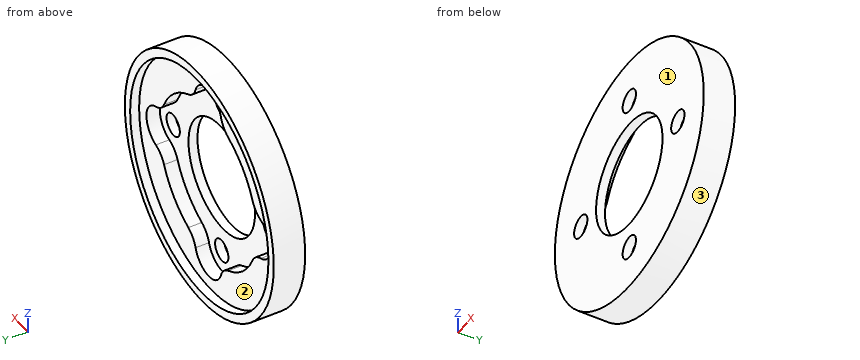
from build123d import *

# Parameters (mm, degrees)
SKETCH1_R           = 28
SKETCH1_R_2         = 12.5
SKETCH1_R_3         = 2.5
BOSS_EXTRUDE1_DEPTH = 5
SKETCH2_R           = 28
SKETCH2_R_2         = 26
BOSS_EXTRUDE2_DEPTH = 2
CUT_EXTRUDE1_DEPTH  = 3
FILLET1_R           = 5


with BuildPart() as part:
    # Sketch1 → Boss-Extrude1 (new body)
    with BuildSketch(Plane(origin=(0, 0, 0), x_dir=(1, 0, 0), z_dir=(0, 1, 0))):
        with Locations(Location((0, 0, 0), (0, 0, 270))):
            Circle(SKETCH1_R)
        with Locations(Location((0, 0, 0), (0, 0, 270))):
            Circle(SKETCH1_R_2, mode=Mode.SUBTRACT)
        with Locations(Location((18.25, 0, 0), (0, 0, 270))):
            Circle(SKETCH1_R_3, mode=Mode.SUBTRACT)
        with Locations(Location((0, -18.25, 0), (0, 0, 270))):
            Circle(SKETCH1_R_3, mode=Mode.SUBTRACT)
        with Locations(Location((-18.25, 0, 0), (0, 0, 270))):
            Circle(SKETCH1_R_3, mode=Mode.SUBTRACT)
        with Locations(Location((0, 18.25, 0), (0, 0, 270))):
            Circle(SKETCH1_R_3, mode=Mode.SUBTRACT)
    extrude(amount=BOSS_EXTRUDE1_DEPTH)

    # Sketch2 → Boss-Extrude2 (add)
    with BuildSketch(Plane(origin=(0, 5, 0), x_dir=(1, 0, 0), z_dir=(0, 1, 0))):
        with Locations(Location((0, 0, 0), (0, 0, 270))):
            Circle(SKETCH2_R)
        with Locations(Location((0, 0, 0), (0, 0, 270))):
            Circle(SKETCH2_R_2, mode=Mode.SUBTRACT)
    extrude(amount=BOSS_EXTRUDE2_DEPTH)

    # Sketch4 → Cut-Extrude1 (cut)
    with BuildSketch(Plane(origin=(0, 5, 0), x_dir=(1, 0, 0), z_dir=(0, 1, 0))):
        with BuildLine():
            ThreePointArc((4.95286471, 17.565068493), (0, 23.25), (-4.95286471, 17.565068493))
            ThreePointArc((-4.95286471, 17.565068493), (-12.904698757, 12.904698757), (-17.565068493, 4.95286471))
            ThreePointArc((-17.565068493, 4.95286471), (-23.25, 0), (-17.565068493, -4.95286471))
            ThreePointArc((-17.565068493, -4.95286471), (-12.904698757, -12.904698757), (-4.95286471, -17.565068493))
            ThreePointArc((-4.95286471, -17.565068493), (0, -23.25), (4.95286471, -17.565068493))
            ThreePointArc((4.95286471, -17.565068493), (12.904698757, -12.904698757), (17.565068493, -4.95286471))
            ThreePointArc((17.565068493, -4.95286471), (23.25, 0), (17.565068493, 4.95286471))
            ThreePointArc((17.565068493, 4.95286471), (12.904698757, 12.904698757), (4.95286471, 17.565068493))
        make_face()
    extrude(amount=-CUT_EXTRUDE1_DEPTH, mode=Mode.SUBTRACT)

    # Fillet1
    fillet1_edges = [part.edges().sort_by_distance(p)[0] for p in [
        (-4.95286471, 3.5, 17.565068493),
        (-17.565068493, 3.5, 4.95286471),
        (-17.565068493, 3.5, -4.95286471),
        (-4.95286471, 3.5, -17.565068493),
        (4.95286471, 3.5, -17.565068493),
        (17.565068493, 3.5, -4.95286471),
        (17.565068493, 3.5, 4.95286471),
        (4.95286471, 3.5, 17.565068493),
    ]]
    fillet(fillet1_edges, radius=FILLET1_R)


solid = part.part
CAD build for the part. Positions are in the model's coordinates, mm. Face numbers are marked on the shaded views. Round coordinates to 2 decimals unless told otherwise and drop trailing zeros. Order: outer loops, then holes, each group sorted by start corner. A loop starts at its lowest first (then second) coordinate and runs counter-clockwise, first axis right, second up. Notation, with made-up numbers: (-13.5, -39.75) -> (18.5, -39.75) arc R27 cw to (18.5, -0.75) -> close; hole circle Ø5 at (70, 11.5). An arc over 180 degrees is marked (long way). Write item = value, one per line. Start each with the question number.
(1) Pull direction X, two halves, no side cores. Call the marked faces 1, 2 and 3: released by +X, released by -X, zero draft, split by the parting line, or undercut.
(2) Cut at D-D, the plane x = -9. List the corners of the cut face in (y, z), then the cut area to 3 significant figures.
(3) Probe line 1 (X direction, y = 1.65, z = 0); line 2 (X direction, y = 1.25, z = -1.5); line 3 (Y direction, x = 20, z = -3.5). List the from-to ranges inside material, lowest first. Write a range as [from, to].
(4) Cut at B-B, the plane x = 0. List the corners of the cut face in (y, z), then the cut area to 3 significant figures.
(5) Cut at A-A, the plane z = 0. List the corners of the cut face in (x, y), then the cut area to 3 significant figures.
(6) Cut at C-C, the plane y = 0.75. List the corners of the cut face in (x, z).
(7) Pin check, flat tips, straight feed: P1, Ø4.5, axis at x = 18.25, z = 0, coming from the +Y side; P2, Ø4, axis at y = 3.5, z = -11, coming from the -X side; P3, Ø8, axis at x = 0, z = 18.25, coming from the +Y side; P4, Ø4, axis at x = -11.5, y = 4, coming from the -Z side. Stop position of each tip, or through.
Model answer:
q1.face_1 = zero draft
q1.face_2 = undercut
q1.face_3 = split by the parting line
q2.outline = (0, -26.51) -> (7, -26.51) -> (7, -24.39) -> (5, -24.39) -> (5, -15.88) -> (2, -15.88) -> (2, -8.67) -> (0, -8.67) -> close; (0, 8.67) -> (2, 8.67) -> (2, 15.88) -> (5, 15.88) -> (5, 24.39) -> (7, 24.39) -> (7, 26.51) -> (0, 26.51) -> close
q2.area = 144 mm2
q3.line_1 = [-28, -20.75], [-15.75, -12.5], [12.5, 15.75], [20.75, 28]
q3.line_2 = [-27.96, -20.25], [-16.25, -12.41], [12.41, 16.25], [20.25, 27.96]
q3.line_3 = [0, 2]
q4.outline = (0, -28) -> (7, -28) -> (7, -26) -> (5, -26) -> (5, -23.25) -> (2, -23.25) -> (2, -20.75) -> (0, -20.75) -> close; (0, -15.75) -> (2, -15.75) -> (2, -12.5) -> (0, -12.5) -> close; (0, 12.5) -> (2, 12.5) -> (2, 15.75) -> (0, 15.75) -> close; (0, 20.75) -> (2, 20.75) -> (2, 23.25) -> (5, 23.25) -> (5, 26) -> (7, 26) -> (7, 28) -> (0, 28) -> close
q4.area = 78.5 mm2
q5.outline = (-28, 0) -> (-20.75, 0) -> (-20.75, 2) -> (-23.25, 2) -> (-23.25, 5) -> (-26, 5) -> (-26, 7) -> (-28, 7) -> close; (-15.75, 0) -> (-12.5, 0) -> (-12.5, 2) -> (-15.75, 2) -> close; (12.5, 0) -> (15.75, 0) -> (15.75, 2) -> (12.5, 2) -> close; (20.75, 0) -> (28, 0) -> (28, 7) -> (26, 7) -> (26, 5) -> (23.25, 5) -> (23.25, 2) -> (20.75, 2) -> close
q5.area = 78.5 mm2
q6.outline = circle Ø56 at (0, 0); hole circle Ø5 at (-18.25, 0); hole circle Ø25 at (0, 0); hole circle Ø5 at (0, -18.25); hole circle Ø5 at (0, 18.25); hole circle Ø5 at (18.25, 0)
q7.P1 = through
q7.P2 = -26.51
q7.P3 = 2
q7.P4 = -26.34
